Check sheet for the modelled part. Datum: model origin and axes. Units: mm. Give positions to 0.01 mm unless a question says otherwise; leave off trailing zeros. Loops run counter-clockwise (first coordinate to the right, second up) from the corner with the lowest first, then second, coordinate; pieces in that order, holes last. Notation, with made-up numbers: (43, 53.5) -> (51, 53.5) arc R21 cw to (51, 65.5) -> close; hole circle Ø6 at (34.5, 72). An arc over 180 degrees is marked (long way). Write each question's results on one line, items separated by ' | '. Start each with the question number.
1. Cross-section at B-B on x = 0. Record the boundary of the cut face in (y, z).
2. Mould release check, pull along X, two halves, no side actions. Record for faces 1 (the face through (-3.4, -12.3, 11.6)), 2 (the face through (-12.488, 0.55, 186.898)), 3 (the face through (-14.985, 0.66, 190.125)): +X half, -X half, draft (parallel to the pull), parting line (faces both ways), or undercut.
3. Material ranges on L1, parallel to Y at x = 0, z = 121; L2, parallel to X at y = -2, z = 138, recorded low to high. Write a range as from..to.
4. Cross-section at C-C on z = 340. Record the boundary of the cut face in (x, y), and give its area (3 significant figures).
5. Gauge pin test, flat ends, axial feed: pin 1 Ø3 at (x, y) = (9, 5) entering from -Z; pin 2 Ø4 at (x, z) = (10.5, 319.5) entering from -Y; pin 3 Ø1 at (y, z) = (0.5, 280) entering from +X; pin 4 Ø2 at (y, z) = (-2.5, 150) entering from -X. Record the tip position at first contact, or that the pin passes through.
6. Cross-section at A-A on y = 0. Record the boundary of the cut face in (x, z).
from build123d import *

# Parameters (mm, degrees)
SKETCH_2_R               = 15
SKETCH_3_R               = 12.5
CUT_EXTRUDE_1_DEPTH      = 376.599520766
CUT_EXTRUDE_2_DEPTH      = 376.599520766
CUT_EXTRUDE_2_DEPTH_BACK = 376.599520766
CUT_EXTRUDE_4_DEPTH      = 376.599520766
CUT_EXTRUDE_4_DEPTH_BACK = 376.599520766


with BuildPart() as part:
    # По траектории1: sweep along a path in Эскиз1
    with BuildLine(Plane(origin=(0, 0, 0), x_dir=(1, 0, 0), z_dir=(0, 1, 0))) as sweep_1_path:
        Line((0, 0), (0, -375))
    # Эскиз2 → По траектории1 (sweep)
    with BuildSketch(Plane.XY):
        Circle(SKETCH_2_R)
    sweep(path=sweep_1_path.line)

    # Эскиз3 → Вырез-Вытянуть1 (cut, through all)
    with BuildSketch(Plane.XY.offset(375)):
        Circle(SKETCH_3_R)
    extrude(amount=-CUT_EXTRUDE_1_DEPTH, mode=Mode.SUBTRACT)

    # Эскиз4 → Вырез-Вытянуть2 (cut, two sides: drawn at the far end of the back side and taken through both)
    with BuildSketch(Plane(origin=(0, 0, 0), x_dir=(1, 0, 0), z_dir=(0, 1, 0)).offset(-CUT_EXTRUDE_2_DEPTH_BACK)):
        Polygon((-15, 0), (15, -30), (15, 0), align=None)
    extrude(amount=CUT_EXTRUDE_2_DEPTH + CUT_EXTRUDE_2_DEPTH_BACK, mode=Mode.SUBTRACT)

    # Эскиз5 → Вырез-Вытянуть4 (cut, two sides: drawn at the far end of the back side and taken through both)
    with BuildSketch(Plane(origin=(0, 0, 0), x_dir=(0, 0, -1), z_dir=(1, 0, 0)).offset(-CUT_EXTRUDE_4_DEPTH_BACK)):
        with BuildLine():
            Line((-375, 15), (-375, -15))
            ThreePointArc((-375, -15), (-360, 0), (-375, 15))
        make_face()
    extrude(amount=CUT_EXTRUDE_4_DEPTH + CUT_EXTRUDE_4_DEPTH_BACK, mode=Mode.SUBTRACT)


solid = part.part
Geometry says:
1) outline: (-15, 15) -> (-12.5, 15) -> (-12.5, 366.71) arc R15 cw to (-15, 375) -> close; (12.5, 15) -> (15, 15) -> (15, 375) arc R15 cw to (12.5, 366.71) -> close
2) face 1: +X half | face 2: undercut | face 3: parting line
3) L1: -15..-12.5, 12.5..15 | L2: -14.87..-12.34, 12.34..14.87
4) outline: circle Ø30 at (0, 0); hole circle Ø25 at (0, 0) | area: 216 mm^2
5) pin 1: through | pin 2: y = -12.36 | pin 3: x = 15 | pin 4: x = -14.92
6) outline: (-15, 0) -> (-12.5, 2.5) -> (-12.5, 360) -> (-15, 360) -> close; (12.5, 27.5) -> (15, 30) -> (15, 360) -> (12.5, 360) -> close
